Verification items for the finished model (mm, model axes). Round coordinates to 2 decimals unless told otherwise and drop trailing zeros. Order: outer loops, then holes, each group sorted by start corner. A loop starts at its lowest first (then second) coordinate and runs counter-clockwise, first axis right, second up. Notation, with made-up numbers: M -18,-31.75 L -8,-31.75 A18 ccw -8,-15.75 Z; hole C 17,-23 d10. An arc over 180 degrees is marked long. Return JSON: item names as keys, results as strings. Group by question number.
from build123d import *

# Parameters (mm, degrees)
CROQUIS1_R              = 31.5
SALIENTE_EXTRUIR1_DEPTH = 3.6
CROQUIS2_R              = 1.5
CORTAR_EXTRUIR1_DEPTH   = 3.6
CROQUIS3_R              = 3
CORTAR_EXTRUIR2_DEPTH   = 2
CROQUIS4_W              = 15
CROQUIS4_H              = 25
SALIENTE_EXTRUIR2_DEPTH = 3
SALIENTE_EXTRUIR4_DEPTH = 25
CORTAR_EXTRUIR6_DEPTH   = 23


with BuildPart() as part:
    # Croquis1 → Saliente-Extruir1 (new body)
    with BuildSketch(Plane.XY):
        with Locations((-75.665270593, 11.323426573)):
            Circle(CROQUIS1_R)
    extrude(amount=SALIENTE_EXTRUIR1_DEPTH)

    # Croquis2 → Cortar-Extruir1 (cut)
    with BuildSketch(Plane.XY.offset(3.6)):
        with Locations((-92.282279951, 27.940435931)):
            Circle(CROQUIS2_R)
        with Locations((-59.048261236, 27.940435931)):
            Circle(CROQUIS2_R)
        with Locations((-59.048261236, -5.293582784)):
            Circle(CROQUIS2_R)
        with Locations((-92.282279951, -5.293582784)):
            Circle(CROQUIS2_R)
    extrude(amount=-CORTAR_EXTRUIR1_DEPTH, mode=Mode.SUBTRACT)

    # Croquis3 → Cortar-Extruir2 (cut)
    with BuildSketch(Plane.XY.offset(3.6)):
        with Locations((-92.282279951, 27.940435931)):
            Circle(CROQUIS3_R)
        with Locations((-59.048261236, 27.940435931)):
            Circle(CROQUIS3_R)
        with Locations((-59.048261236, -5.293582784)):
            Circle(CROQUIS3_R)
        with Locations((-92.282279951, -5.293582784)):
            Circle(CROQUIS3_R)
    extrude(amount=-CORTAR_EXTRUIR2_DEPTH, mode=Mode.SUBTRACT)

    # Croquis4 → Saliente-Extruir2 (add)
    with BuildSketch(Plane.XY.offset(3.6)):
        with Locations((-75.665270593, 11.323426573)):
            Rectangle(CROQUIS4_W, CROQUIS4_H)
    extrude(amount=SALIENTE_EXTRUIR2_DEPTH)

    # Croquis7 → Saliente-Extruir4 (add)
    with BuildSketch(Plane.XZ.offset(1.176573427)):
        Polygon((-83.165270593, 6.6), (-86.165270593, 3.6), (-83.165270593, 3.6), align=None)
        Polygon((-68.165270593, 6.6), (-65.165270593, 3.6), (-68.165270593, 3.6), align=None)
    extrude(amount=-SALIENTE_EXTRUIR4_DEPTH)

    # Croquis8 → Cortar-Extruir6 (cut)
    with BuildSketch(Plane.XZ.offset(1.176573427)):
        Polygon((-83.165270593, 3.6), (-80.165270593, 6.6), (-71.165270593, 6.6), (-68.165270593, 3.6), align=None)
    extrude(amount=-CORTAR_EXTRUIR6_DEPTH, mode=Mode.SUBTRACT)


solid = part.part
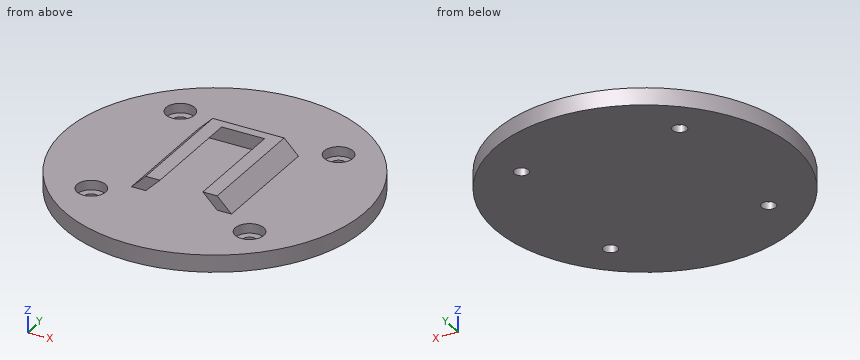
1. Cross-section at A-A (x = -58.5). Enter the section's corners in (y, z).
2. Cross-section at B-B (z = 4.5). Enter the section's corners in (x, y), plus the area to 3 significant figures.
3. Cross-section at D-D (x = -85). Enter the section's corners in (y, z), plus the area to 3 significant figures.
4. Go/stop test with flat-tipped pins: pin 1 (8 mm diameter, centred on x = -92.28, y = -5.29, fed in from +Z); pin 2 (5 mm diameter, centred on x = -59.05, y = -5.29, fed in from +Z); pin 3 (2.5 mm diameter, centred on x = -68, z = 5, fed in from -Y); pin 4 (3 mm diameter, centred on x = -87.5, z = 6, fed in from +Y). Record where each tip stops, or that it passes through.
5. Thickness scan on line 1 along X through (y, z) = (-6.5, 2) (3 decimals); line 2 along X through (y, z) = (29, 0.75); line 3 along Z through (x, y) = (-77, -15.5). Record the ranges inside material, lowest first. Write a range as from..to.
6. Cross-section at C-C (y = 6). Enter the section's corners in (x, z), plus the area to 3 significant figures.
Computed:
{
 "1": {"outline": "M -15.09,0 L -6.69,0 L -6.69,1.6 L -8.24,1.6 L -8.24,3.6 L -15.09,3.6 Z; M -3.9,0 L 26.54,0 L 26.54,1.6 L 24.99,1.6 L 24.99,3.6 L -2.34,3.6 L -2.34,1.6 L -3.9,1.6 Z; M 29.34,0 L 37.74,0 L 37.74,3.6 L 30.89,3.6 L 30.89,1.6 L 29.34,1.6 Z"},
 "2": {"outline": "M -85.27,-1.18 L -82.27,-1.18 L -82.27,21.82 L -69.07,21.82 L -69.07,-1.18 L -66.07,-1.18 L -66.07,23.82 L -85.27,23.82 Z", "area": "176 mm²"},
 "3": {"outline": "M -18.76,0 L 41.41,0 L 41.41,3.6 L 23.82,3.6 L 23.82,4.77 L -1.18,4.77 L -1.18,3.6 L -18.76,3.6 Z", "area": "246 mm²"},
 "4": {"pin 1": "stops at z = 3.6", "pin 2": "stops at z = 1.6", "pin 3": "stops at y = -1.18", "pin 4": "passes through"},
 "5": {"line 1": "x = -101.638..-95.029, -89.536..-61.795, -56.302..-49.693", "line 2": "x = -101.74..-93.34, -91.22..-60.11, -57.99..-49.59", "line 3": "z = 0..3.6"},
 "6": {"outline": "M -106.71,0 L -44.62,0 L -44.62,3.6 L -65.17,3.6 L -68.17,6.6 L -71.17,6.6 L -68.17,3.6 L -83.17,3.6 L -80.17,6.6 L -83.17,6.6 L -86.17,3.6 L -106.71,3.6 Z", "area": "242 mm²"}
}
